```python
from build123d import *

# Parameters (mm, degrees)
BOSS_EXTRUDE1_DEPTH = 0.5953125
SKETCH2_R           = 0.5953125
BOSS_EXTRUDE2_DEPTH = 22.225


with BuildPart() as part:
    # Sketch1 → Boss-Extrude1 (new, symmetric)
    with BuildSketch(Plane.XY):
        Polygon((-18.25625, 0), (18.25625, 0), (18.25625, 19.05), (21.43125, 19.05), (21.43125, 44.45), (-21.43125, 44.45), (-21.43125, 19.05), (-18.25625, 19.05), align=None)
    extrude(amount=BOSS_EXTRUDE1_DEPTH, both=True)

    # Sketch2 → Boss-Extrude2 (add, symmetric)
    with BuildSketch(Plane(origin=(0, 0, 0), x_dir=(0, 0, -1), z_dir=(1, 0, 0))):
        with Locations((0, 3.571875)):
            Circle(SKETCH2_R)
    extrude(amount=BOSS_EXTRUDE2_DEPTH, both=True)


solid = part.part
```
Work out the finished part from the listing and answer in its coordinate system (mm). A direction names the side the tool comes from. Give positions to 0.01 mm unless a question says otherwise; leave off trailing zeros. Order: outer loops, then holes, each group sorted by start corner. A loop starts at its lowest first (then second) coordinate and runs counter-clockwise, first axis right, second up. Notation, with made-up numbers: (-27.5, -21) - (31.5, -21) arc R24 ccw to (31.5, -5) - close; hole circle Ø1 at (34.5, 82). An arc over 180 degrees is marked (long way). One line per item, written item: value. Start each with the question number.
1. Section B-B, the plane y = 8 is taken. Write down the section's boundary in (x, z).
2. Section C-C, the plane y = 42 is taken. Write down the section's boundary in (x, z).
3. Which of the six approach directions +Z, -Z, +X, -X, +Y, -Y give full straight-line access (tool end or side, diameter ignored) to faces 1 (the face through (21.431, 32, 0)), 2 (the face through (-20, 19.05, 0)), 3 (the face through (20, 19.05, 0)), 4 (the face through (-21.431, 32, 0))?
4. Each of these flat-tipped pins is pushed along its axis until it touches: pin 1 Ø0.6 at (y, z) = (9.5, 0) entering from +X; pin 2 Ø0.6 at (y, z) = (1.5, 0) entering from -X. Where does it stop, or does it pass through?
5. For a pull along Y with two mould halves and no side action, classify faces 5 (the face through (0, 0, 0)), 6 (the face through (-20.21, 2.99, 0.13)), 7 (the face through (18.256, 11, 0)), 8 (the face through (-22.225, 4, 0)) as released by +Y, released by -Y, zero draft, split by the parting line, or undercut.
6. Consider line 1 (X direction, y = 24, z = 0.4); line 2 (X direction, y = 9, z = 0.3). Determine where each line is inside the solid, lowest interval first.
7. Section A-A, the plane z = 0 is taken. Write down the section's boundary in (x, y) (3 decimals).
Filled sheet:
1. outline: (-18.26, -0.6) - (18.26, -0.6) - (18.26, 0.6) - (-18.26, 0.6) - close
2. outline: (-21.43, -0.6) - (21.43, -0.6) - (21.43, 0.6) - (-21.43, 0.6) - close
3. face 1: +Z, -Z, +X, +Y
3. face 2: +Z, -Z, -X
3. face 3: +Z, -Z, +X
3. face 4: +Z, -Z, -X, +Y
4. pin 1: x = 18.26
4. pin 2: x = -18.26
5. face 5: released by -Y
5. face 6: undercut
5. face 7: undercut
5. face 8: zero draft
6. line 1: -21.43 to 21.43
6. line 2: -18.26 to 18.26
7. outline: (-22.225, 2.977) - (-18.256, 2.977) - (-18.256, 0) - (18.256, 0) - (18.256, 2.977) - (22.225, 2.977) - (22.225, 4.167) - (18.256, 4.167) - (18.256, 19.05) - (21.431, 19.05) - (21.431, 44.45) - (-21.431, 44.45) - (-21.431, 19.05) - (-18.256, 19.05) - (-18.256, 4.167) - (-22.225, 4.167) - close
